```python
from build123d import *

# Parameters (mm, degrees)
SKETCH1_W           = 61.3
SKETCH1_H           = 25.4
BOSS_EXTRUDE1_DEPTH = 5.334
SKETCH2_W           = 2.4638
SKETCH2_H           = 6.35
SKETCH2_W_2         = 5.334
CUT_EXTRUDE1_DEPTH  = 67.568022023


with BuildPart() as part:
    # Sketch1 → Boss-Extrude1 (new body)
    with BuildSketch(Plane(origin=(0, 0, 0), x_dir=(0, 0, -1), z_dir=(1, 0, 0))):
        with Locations((30.65, 12.7)):
            Rectangle(SKETCH1_W, SKETCH1_H)
    extrude(amount=BOSS_EXTRUDE1_DEPTH)

    # Sketch2 → Cut-Extrude1 (cut, through all)
    with BuildSketch(Plane(origin=(5.334, 0, 0), x_dir=(0, 0, -1), z_dir=(1, 0, 0))):
        with Locations((1.2319, 22.225)):
            Rectangle(SKETCH2_W, SKETCH2_H)
        with Locations((1.2319, 3.175)):
            Rectangle(SKETCH2_W, SKETCH2_H)
        with Locations((23.1308, 22.225)):
            Rectangle(SKETCH2_W_2, SKETCH2_H)
        with Locations((23.1308, 3.175)):
            Rectangle(SKETCH2_W_2, SKETCH2_H)
        with Locations((58.633, 3.175)):
            Rectangle(SKETCH2_W_2, SKETCH2_H)
        with Locations((58.633, 22.225)):
            Rectangle(SKETCH2_W_2, SKETCH2_H)
    extrude(amount=-CUT_EXTRUDE1_DEPTH, mode=Mode.SUBTRACT)


solid = part.part
```
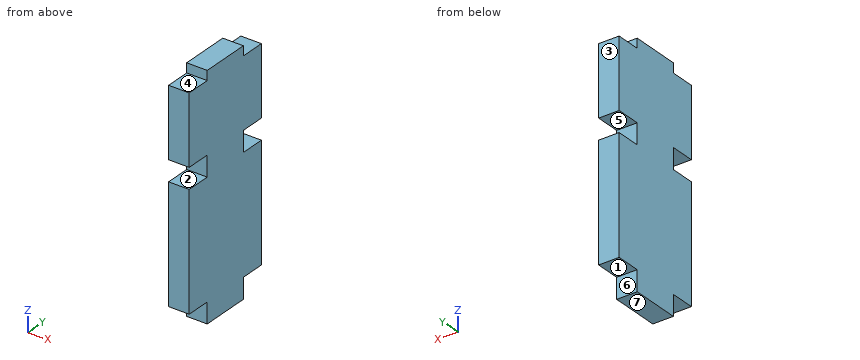
Input: part model. Units: mm. Frame: model coordinates. Face numbers are marked on the shaded views. A direction names the side the tool comes from. Coordinates: 2 decimals unless noted, no trailing zeros. Write each loop counter-clockwise with the first axis right and the second up, starting at its lowest first coordinate (ties: lowest second). Pieces come first, ordered by that corner, then holes. Notation, with made-up numbers: M -21,38 L 5,38 A22 ccw 5,70 Z; hole C 78.5,4.25 d2. An arc over 180 degrees is marked long. Use one line per item in the form item = value.
Q1. First-contact query: pin 1 (1.6 mm diameter, centred on x = 2, y = 3.5, fed in from -Z); pin 2 (2.5 mm diameter, centred on x = 2.5, z = -58, fed in from +Y); pin 3 (1.6 mm diameter, centred on x = 1.5, y = 22, fed in from +Z). Flat tips, straight axial feed; report the tip coordinate or a pass-through.
Answer below:
pin_1 = -55.97
pin_2 = 19.05
pin_3 = -2.46
Q2. Section B-B (x = 4.55). Return loops of the section in (y, z), plus the area to 3 significant figures.
Answer below:
outline = M 0,-55.97 L 6.35,-55.97 L 6.35,-61.3 L 19.05,-61.3 L 19.05,-55.97 L 25.4,-55.97 L 25.4,-25.8 L 19.05,-25.8 L 19.05,-20.46 L 25.4,-20.46 L 25.4,-2.46 L 19.05,-2.46 L 19.05,0 L 6.35,0 L 6.35,-2.46 L 0,-2.46 L 0,-20.46 L 6.35,-20.46 L 6.35,-25.8 L 0,-25.8 Z
area = 1,390 mm²
Q3. Section C-C (z = -23). Return loops of the section in (x, y).
Answer below:
outline = M 0,6.35 L 5.33,6.35 L 5.33,19.05 L 0,19.05 Z
Q4. Draft query along Z for the marked faces 4, 5, 6 and 7. Return one class per face: released by +Z, released by -Z, zero draft, split by the parting line, or undercut.
Answer below:
face_4 = released by +Z
face_5 = undercut
face_6 = zero draft
face_7 = released by -Z
Q5. Set-up query: the marked faces 1, 2 and 3. Return all of +Z, -Z, +X, -X, +Y, -Y with unobstructed straight access to the full face (end or side cutting, diameter ignored); none if empty.
Answer below:
face_1 = -Z, +X, -X, +Y
face_2 = +X, -X, -Y
face_3 = +Z, -Z, +X, -X, +Y
Q6. Section A-A (y = 21). Return loops of the section in (x, z), plus the area to 3 significant figures.
Answer below:
outline = M 0,-55.97 L 5.33,-55.97 L 5.33,-25.8 L 0,-25.8 Z; M 0,-20.46 L 5.33,-20.46 L 5.33,-2.46 L 0,-2.46 Z
area = 257 mm²
Q7. Material intervals for probe 1 along Z at (x, y) = (4.05, 3.25); probe 2 along Y at (x, z) = (2.5, -20.5), sorted ascending. Write a range as from..to.
Answer below:
probe_1 = -55.97..-25.8, -20.46..-2.46
probe_2 = 6.35..19.05
